Work out the finished part from the listing and answer in its coordinate system (mm). Round coordinates to 2 decimals unless told otherwise and drop trailing zeros. Order: outer loops, then holes, each group sorted by start corner. A loop starts at its lowest first (then second) coordinate and runs counter-clockwise, first axis right, second up. Notation, with made-up numbers: (12, 39) -> (32, 39) arc R12 cw to (32, 46) -> close; hole circle Ø9 at (70, -19). An arc over 180 degrees is marked (long way). Use a Markdown table: item, result. Add a question column.
Item 1: A cutting plane is placed at A-A, the plane x = 11359.5. Determine the outline of the cut face in (y, z).
Item 2: A cutting plane is placed at B-B, the plane y = -4828.5. Determine the outline of the cut face in (x, z), plus the area to 3 significant figures.
Item 3: Find the intervals of material crossed by L1, parallel to X at y = -5212, z = -4.5 (3 decimals); L2, parallel to Y at x = 11744.5, z = -2.75; L3, parallel to X at y = -5093.5, z = -8.25, in increasing order. Write a range as [from, to].
Item 4: For a pull along X with two mould halves and no side action, classify faces 1 (the flat face through (11591, -5018, -17.78)), 2 (the cylindrical face through (11026.116, -4877.357, -8.766)), 3 (the flat face through (11519.625, -4754.864, -8.766)) as +X half, -X half, draft (parallel to the pull), parting line (faces both ways), or undercut.
Item 5: Flat-ended cylindrical pins translate along their axes: P1, Ø3, axis at x = 10955.23, y = -4929.98, coming from the -Z side; P2, Ø1.5, axis at y = -5195.5, z = -2, coming from the +X side; P3, Ø8, axis at x = 11222.5, z = -10, coming from the +Y side; P4, Ø8, axis at x = 11273.5, z = -2.5, coming from the +Y side. Find the tip coordinate at first contact, or state that the pin passes through.
Item 6: A cutting plane is placed at C-C, the plane x = 11560.5. Determine the outline of the cut face in (y, z), plus the area to 3 significant figures.
from build123d import *

# Parameters (mm, degrees)
CABSIDELEFT_THICKNESS_DEPTH = 17.78
LEDGECUTS_DEPTH_DEPTH       = 5.08
CABFRONTLEDGECUT_W          = 17.78
CABFRONTLEDGECUT_H          = 402.324113577
FRONTLEDGECUT_DEPTH_DEPTH   = 11.43
SKETCH5_R                   = 15.08125
SKETCH5_R_2                 = 1.5875
CUT_EXTRUDE3_DEPTH          = 17.78
SKETCH6_R                   = 3.302
CUT_EXTRUDE4_DEPTH          = 5.08
CUT_EXTRUDE5_DEPTH          = 594.36
SKETCH8_R                   = 2.38125
CUT_EXTRUDE6_DEPTH          = 17.78
SKETCH9_R                   = 1.5875
CUT_EXTRUDE7_DEPTH          = 12.7
SKETCH10_R                  = 4.7625
CUT_EXTRUDE8_DEPTH          = 76.2
SKETCH11_R                  = 4.7625
CUT_EXTRUDE9_DEPTH          = 76.2


with BuildPart() as part:
    # CabSideLeft_Outline → CabSideLeft_Thickness (new body)
    with BuildSketch(Plane.XY):
        Polygon((10946.341666666, -4853.78125), (10946.341666666, -5253.0375), (12254.441666666, -5253.0375), (12254.441666666, -4658.6775), (12077.077955444, -4658.6775), align=None)
    extrude(amount=-CABSIDELEFT_THICKNESS_DEPTH)

    # CabSideLeft_LedgeCuts → LedgeCuts_Depth (cut)
    with BuildSketch(Plane.XY):
        Polygon((10946.341666666, -5225.7325), (10946.341666666, -5243.5125), (12236.661666666, -5243.5125), (12236.661666666, -5253.0375), (12254.441666666, -5253.0375), (12254.441666666, -4658.6775), (12236.661666666, -4658.6775), (12236.661666666, -5225.7325), (11824.335, -5225.7325), (11824.335, -5141.9125), (11806.555, -5141.9125), (11806.555, -5225.7325), (11394.228333334, -5225.7325), (11394.228333334, -5141.912499999), (11376.448333334, -5141.9125), (11376.448333334, -5225.7325), align=None)
    extrude(amount=-LEDGECUTS_DEPTH_DEPTH, mode=Mode.SUBTRACT)

    # CabFrontLedgeCut → FrontLedgeCut_Depth (cut)
    with BuildSketch(Plane.XY):
        with Locations((10955.231666666, -5051.875443212)):
            Rectangle(CABFRONTLEDGECUT_W, CABFRONTLEDGECUT_H)
    extrude(amount=-FRONTLEDGECUT_DEPTH_DEPTH, mode=Mode.SUBTRACT)

    # Sketch5 → Cut-Extrude3 (cut)
    with BuildSketch(Plane.XY):
        with Locations((11037.231463428, -4887.549352662)):
            Circle(SKETCH5_R)
        with Locations((11003.796466666, -5033.9625)):
            Circle(SKETCH5_R_2)
        with Locations((10955.231666666, -4929.98125)):
            Circle(SKETCH5_R_2)
        with Locations((10955.231666666, -5031.58125)):
            Circle(SKETCH5_R_2)
        with Locations((11003.809166666, -5062.5375)):
            Circle(SKETCH5_R_2)
        with Locations((11003.809166666, -5119.6875)):
            Circle(SKETCH5_R_2)
        with Locations((11003.809166666, -5176.8375)):
            Circle(SKETCH5_R_2)
        with Locations((11251.141666666, -5234.6225)):
            Circle(SKETCH5_R_2)
        with Locations((11098.741666666, -5234.6225)):
            Circle(SKETCH5_R_2)
        with Locations((11385.338333334, -5160.9625)):
            Circle(SKETCH5_R_2)
        with Locations((11385.338333334, -5193.9825)):
            Circle(SKETCH5_R_2)
        with Locations((11530.541666666, -5234.6225)):
            Circle(SKETCH5_R_2)
        with Locations((11682.941666666, -5234.6225)):
            Circle(SKETCH5_R_2)
        with Locations((11815.445, -5160.9625)):
            Circle(SKETCH5_R_2)
        with Locations((11815.445, -5193.9825)):
            Circle(SKETCH5_R_2)
        with Locations((11962.341666666, -5234.6225)):
            Circle(SKETCH5_R_2)
        with Locations((12114.741666666, -5234.6225)):
            Circle(SKETCH5_R_2)
        with Locations((12196.974166666, -5202.2375)):
            Circle(SKETCH5_R_2)
        with Locations((12196.974166666, -5145.0875)):
            Circle(SKETCH5_R_2)
        with Locations((12245.551666666, -5134.504166666)):
            Circle(SKETCH5_R_2)
        with Locations((12196.974166666, -5087.9375)):
            Circle(SKETCH5_R_2)
        with Locations((12245.551666666, -5015.970833334)):
            Circle(SKETCH5_R_2)
        with Locations((12245.551666666, -4897.4375)):
            Circle(SKETCH5_R_2)
        with Locations((12245.551666666, -4778.904166666)):
            Circle(SKETCH5_R_2)
        with Locations((11003.796466666, -5091.1125)):
            Circle(SKETCH5_R_2)
        with Locations((11003.796466666, -5148.2625)):
            Circle(SKETCH5_R_2)
    extrude(amount=-CUT_EXTRUDE3_DEPTH, mode=Mode.SUBTRACT)

    # Sketch6 → Cut-Extrude4 (cut)
    with BuildSketch(Plane.XY):
        with Locations((11378.693397364, -5144.15756403)):
            Circle(SKETCH6_R)
        with Locations((11391.983269304, -5144.157564029)):
            Circle(SKETCH6_R)
        with Locations((11808.80006403, -5144.15756403)):
            Circle(SKETCH6_R)
        with Locations((11822.08993597, -5144.15756403)):
            Circle(SKETCH6_R)
    extrude(amount=-CUT_EXTRUDE4_DEPTH, mode=Mode.SUBTRACT)

    # FrontBevelCut → Cut-Extrude5 (cut)
    with BuildSketch(Plane.XZ.offset(5253.0375)):
        Polygon((10946.341666666, -17.78), (10946.341666666, -11.43), (10952.691666666, -11.43), align=None)
    extrude(amount=-CUT_EXTRUDE5_DEPTH, mode=Mode.SUBTRACT)

    # Sketch8 → Cut-Extrude6 (cut)
    with BuildSketch(Plane(origin=(0, 0, -17.78), x_dir=(-1, 0, 0), z_dir=(0, 0, -1))):
        with Locations((-10988.502040274, -4864.401180469)):
            Circle(SKETCH8_R)
        with Locations((-12108.60052224, -4671.132938908)):
            Circle(SKETCH8_R)
    extrude(amount=-CUT_EXTRUDE6_DEPTH, mode=Mode.SUBTRACT)

    # Sketch9 → Cut-Extrude7 (cut)
    with BuildSketch(Plane.XY):
        with Locations((12130.320157336, -4901.492108659)):
            Circle(SKETCH9_R)
        with Locations((11939.909008281, -4907.309695425)):
            Circle(SKETCH9_R)
        with Locations((11749.497859227, -4913.127282192)):
            Circle(SKETCH9_R)
    extrude(amount=-CUT_EXTRUDE7_DEPTH, mode=Mode.SUBTRACT)

    # Sketch10 → Cut-Extrude8 (cut)
    with BuildSketch(Plane(origin=(5498.144384557, 0, 5498.144384557), x_dir=(0.707106781, 0, -0.707106781), z_dir=(0.707106781, 0, 0.707106781))):
        with Locations((7752.804780254, -5119.6875)):
            Circle(SKETCH10_R)
        with Locations((7752.804780254, -5176.8375)):
            Circle(SKETCH10_R)
    extrude(amount=-CUT_EXTRUDE8_DEPTH, mode=Mode.SUBTRACT)

    # Sketch11 → Cut-Extrude9 (cut)
    with BuildSketch(Plane(origin=(5498.150734557, 0, 5498.150734557), x_dir=(0.707106781, 0, -0.707106781), z_dir=(0.707106781, 0, 0.707106781))):
        with Locations((7752.795799998, -5091.1125)):
            Circle(SKETCH11_R)
        with Locations((7752.795799998, -5148.2625)):
            Circle(SKETCH11_R)
    extrude(amount=-CUT_EXTRUDE9_DEPTH, mode=Mode.SUBTRACT)


solid = part.part
Reported:
| question | item | result |
|---|---|---|
| 1 | outline | (-5253.04, -17.78) -> (-4782.49, -17.78) -> (-4782.49, 0) -> (-5225.73, 0) -> (-5225.73, -5.08) -> (-5243.51, -5.08) -> (-5243.51, 0) -> (-5253.04, 0) -> close |
| 2 | outline | (11092.86, -17.78) -> (12254.44, -17.78) -> (12254.44, -5.08) -> (12236.66, -5.08) -> (12236.66, 0) -> (11092.86, 0) -> close |
| 2 | area | 20,600 mm² |
| 3 | L1 | [10964.122, 11376.448], [11394.228, 11806.555], [11824.335, 12236.662] |
| 3 | L2 | [-5253.04, -5243.51], [-5225.73, -4716.06] |
| 3 | L3 | [10964.12, 12254.44] |
| 4 | face 1 | draft |
| 4 | face 2 | undercut |
| 4 | face 3 | -X half |
| 5 | P1 | through |
| 5 | P2 | x = 12236.66 |
| 5 | P3 | y = -4805.44 |
| 5 | P4 | y = -4796.64 |
| 6 | outline | (-5253.04, -17.78) -> (-4747.81, -17.78) -> (-4747.81, 0) -> (-5225.73, 0) -> (-5225.73, -5.08) -> (-5243.51, -5.08) -> (-5243.51, 0) -> (-5253.04, 0) -> close |
| 6 | area | 8,890 mm² |
